CAD build for the part. Positions are in the model's coordinates, mm. A direction names the side the tool comes from. Give positions to 0.01 mm unless a question says otherwise; leave off trailing zeros. Write each loop counter-clockwise with the first axis right and the second up, starting at its lowest first coordinate (ties: lowest second). Pieces come first, ordered by that corner, then holes. Notation, with made-up numbers: (72.25, -5.5) - (88.25, -5.5) arc R18 cw to (88.25, 19.5) - close; hole circle Ø3 at (14.25, 78). An arc over 180 degrees is marked (long way). Put each result on its own line as item: value. Start each with the question number.
1. Cut at C-C on z = 43. List the corners of the cut face in (x, y), and give its area (3 significant figures).
2. Cut at A-A on z = 23. List the corners of the cut face in (x, y), and give its area (3 significant figures).
3. Cut at D-D on x = 130. List the corners of the cut face in (y, z).
4. Wall check: line 1 (X direction, y = 18, z = 20.5); line 2 (Z direction, x = 134.5, y = 12); line 3 (X direction, y = 38, z = 32). Give the ranges that are in metal, low to high.
5. Cut at B-B on y = 57. List the corners of the cut face in (x, z).
6. Tool access for faces 5 (the flat face through (120, 33, 12.7)), 6 (the flat face through (244, 33, 12.7)), 7 (the flat face through (183, 33, 12.7)): list every direction of +Z, -Z, +X, -X, +Y, -Y with a clear straight run to the whole face (end or side of a thin tool).
7. Drop flat-ended pins along their axis: pin 1 (23 mm diameter, centred on x = 114, y = 21.5, fed in from +Z); pin 2 (1.5 mm diameter, centred on y = 57.5, z = 42.5, fed in from +X); pin 3 (19 mm diameter, centred on y = 31.5, z = 24, fed in from -X). Give the stop position or say it passes through.
8. Mould opens along X. For faces 1 (the flat face through (134.92, 32, 31)), 2 (the flat face through (193.721, 32, 20)), 3 (the flat face through (173.02, 32, 20)), 4 (the flat face through (258.456, 32, 6)) say: +X half, -X half, draft (parallel to the pull), parting line (faces both ways), or undercut.
from build123d import *

# Parameters (mm, degrees)
F0_W     = 152.4
F0_H     = 76.2
F1_DEPTH = 12.7
F2_W     = 38.1
F2_H     = 38.1
F3_DEPTH = 76.2
F4_W     = 35.56
F4_H     = 38.1
F5_DEPTH = 76.2
F7_DEPTH = 76.2
F9_DEPTH = 76.2


with BuildPart() as f1:
    # F0 (on Top) → F1 (new body)
    with BuildSketch(Plane.XY):
        with Locations((182.255961, 32.827802)):
            Rectangle(F0_W, F0_H)
    extrude(amount=F1_DEPTH)

    # F2 (on face) → F3 (join)
    with BuildSketch(Plane.XZ.offset(5.272198)):
        with Locations((153.970076, 31.75)):
            Rectangle(F2_W, F2_H)
    extrude(amount=-F3_DEPTH)

    # F4 (on face) → F5 (join)
    with BuildSketch(Plane.XZ.offset(5.272198)):
        with Locations((211.501011, 31.75)):
            Rectangle(F4_W, F4_H)
    extrude(amount=-F5_DEPTH)

    # F6 (on face) → F7 (cut)
    with BuildSketch(Plane.XZ.offset(5.272198)):
        Polygon((173.020076, 50.8), (143.86259, 50.8), (173.020076, 26.959093), align=None)
    extrude(amount=-F7_DEPTH, mode=Mode.SUBTRACT)

    # F8 (on face) → F9 (cut)
    with BuildSketch(Plane.XZ.offset(5.272198)):
        Polygon((193.721011, 26.959093), (219.611079, 50.8), (193.721011, 50.8), align=None)
    extrude(amount=-F9_DEPTH, mode=Mode.SUBTRACT)


solid = f1.part
Report:
1. outline: (134.92, -5.27) - (153.4, -5.27) - (153.4, 70.93) - (134.92, 70.93) - close; (211.14, -5.27) - (229.28, -5.27) - (229.28, 70.93) - (211.14, 70.93) - close
1. area: 2,790 mm²
2. outline: (134.92, -5.27) - (173.02, -5.27) - (173.02, 70.93) - (134.92, 70.93) - close; (193.72, -5.27) - (229.28, -5.27) - (229.28, 70.93) - (193.72, 70.93) - close
2. area: 5,610 mm²
3. outline: (-5.27, 0) - (70.93, 0) - (70.93, 12.7) - (-5.27, 12.7) - close
4. line 1: x = 134.92 to 173.02, 193.72 to 229.28
4. line 2: z = 0 to 12.7
4. line 3: x = 134.92 to 166.86, 199.2 to 229.28
5. outline: (106.06, 0) - (258.46, 0) - (258.46, 12.7) - (229.28, 12.7) - (229.28, 50.8) - (219.61, 50.8) - (193.72, 26.96) - (193.72, 12.7) - (173.02, 12.7) - (173.02, 26.96) - (143.86, 50.8) - (134.92, 50.8) - (134.92, 12.7) - (106.06, 12.7) - close
6. face 5: +Z, -X, +Y, -Y
6. face 6: +Z, +X, +Y, -Y
6. face 7: +Z, +Y, -Y
7. pin 1: stops at z = 12.7
7. pin 2: stops at x = 229.28
7. pin 3: stops at x = 134.92
8. face 1: -X half
8. face 2: undercut
8. face 3: undercut
8. face 4: +X half
